For this review, use the dimensioned drawing (mm, ordinates from the lowest corner) and the shaded views. A direction names the side the tool comes from. Round coordinates to 2 decimals unless told otherwise and drop trailing zeros. Write each loop counter-clockwise with the first axis right and the second up, starting at its lowest first coordinate (ties: lowest second). Pieces come first, ordered by that corner, then holes. Notation, with made-up numbers: M -28.5,27 L 25.5,27 A16 cw 25.5,47 Z; hole C 70,28 d10. An arc over 180 degrees is marked long. Answer in a Markdown table with one row per item.
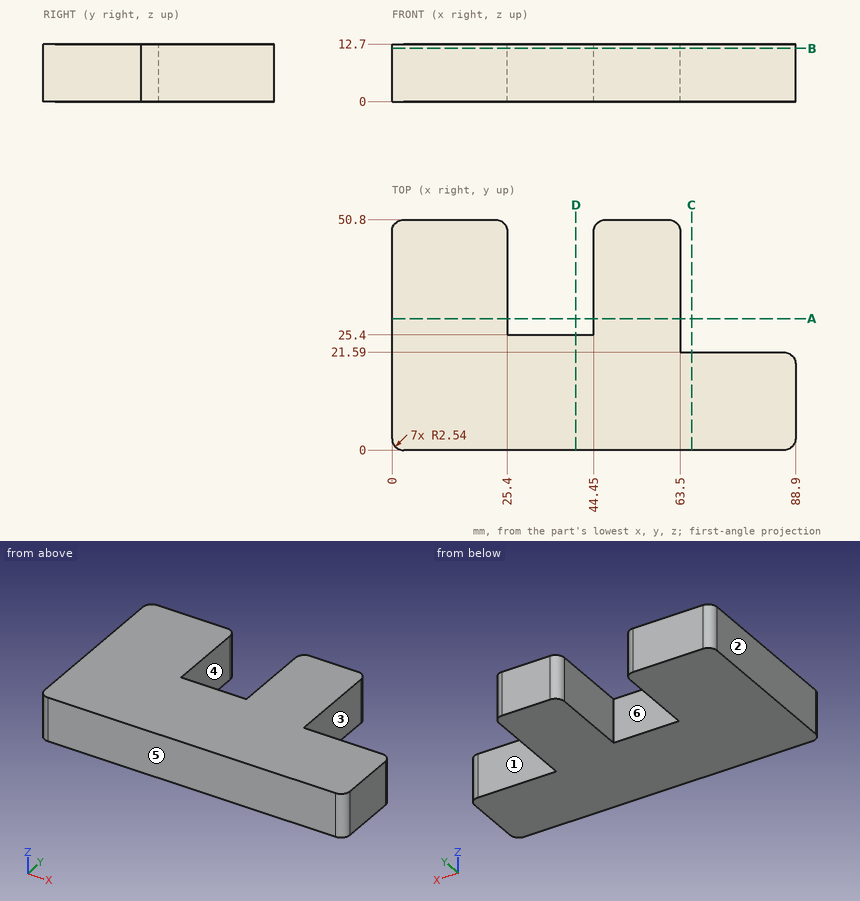
Q1. Take a section at B-B (z = 11.75). State the section outline as (x, y) points, then the cut area to 3 significant figures.
Found:
| item | result |
|---|---|
| outline | M 0,2.54 A2.54 ccw 2.54,0 L 86.36,0 A2.54 ccw 88.9,2.54 L 88.9,19.05 A2.54 ccw 86.36,21.59 L 63.5,21.59 L 63.5,48.26 A2.54 ccw 60.96,50.8 L 46.99,50.8 A2.54 ccw 44.45,48.26 L 44.45,25.4 L 25.4,25.4 L 25.4,48.26 A2.54 ccw 22.86,50.8 L 2.54,50.8 A2.54 ccw 0,48.26 Z |
| area | 3,280 mm² |
Q2. Machinability: for the marked faces 5 and 6, which of the approach directions +Z, -Z, +X, -X, +Y, -Y give a long, thin tool a straight path to every point of the face, cutting with its end or side? Answer none if there is none.
Found:
| item | result |
|---|---|
| face 5 | +Z, -Z, +X, -X, -Y |
| face 6 | +Z, -Z, +Y |
Q3. Take a section at A-A (y = 29). State the section outline as (x, z) points.
Found:
| item | result |
|---|---|
| outline | M 0,0 L 25.4,0 L 25.4,12.7 L 0,12.7 Z; M 44.45,0 L 63.5,0 L 63.5,12.7 L 44.45,12.7 Z |
Q4. Take a section at C-C (x = 66). State the section outline as (y, z) points, then the cut area to 3 significant figures.
Found:
| item | result |
|---|---|
| outline | M 0,0 L 21.59,0 L 21.59,12.7 L 0,12.7 Z |
| area | 274 mm² |
Q5. For probe 1 along X at (y, z) = (29.5, 5); probe 2 along Y at (x, z) = (34, 9); probe 3 along Y at (x, z) = (72, 11), list the stretches that pass through material, from the lowest coordinate up.
Found:
| item | result |
|---|---|
| probe 1 | 0 to 25.4, 44.45 to 63.5 |
| probe 2 | 0 to 25.4 |
| probe 3 | 0 to 21.59 |
Q6. Insertion check: P1, Ø4, axis at x = 79, z = 6.5, coming from the +Y side; P2, Ø6, axis at x = 37.5, z = 2.5, coming from the +Y side. Each pin has a flat end and moves straight along its axis. Give the tip position at first contact, or say it passes through.
Found:
| item | result |
|---|---|
| P1 | y = 21.59 |
| P2 | y = 25.4 |
Q7. Mouldability with a two-part tool opening along X and no side actions: class the marked faces 1, 2, 3 and 4 as +X half, -X half, draft (parallel to the pull), parting line (faces both ways), or undercut.
Found:
| item | result |
|---|---|
| face 1 | draft |
| face 2 | -X half |
| face 3 | +X half |
| face 4 | undercut |
Q8. Take a section at D-D (x = 40.5). State the section outline as (y, z) points, then the cut area to 3 significant figures.
Found:
| item | result |
|---|---|
| outline | M 0,0 L 25.4,0 L 25.4,12.7 L 0,12.7 Z |
| area | 323 mm² |
